For this review, take the finished solid that the model builds, in its own axes (mm). Face numbers are marked on the shaded views. A direction names the side the tool comes from. Coordinates: 2 decimals unless noted, no trailing zeros. Write each loop counter-clockwise with the first axis right and the second up, starting at its lowest first coordinate (ties: lowest second). Pieces come first, ordered by that corner, then holes.
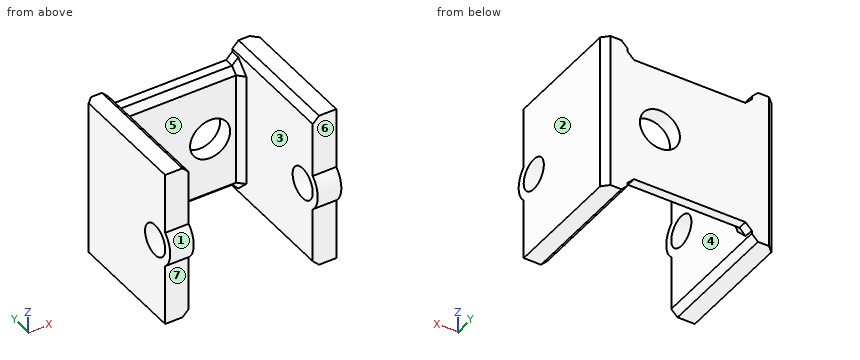
```python
from build123d import *

# Parameters (mm, degrees)
BOSS_EXTRUDE1_DEPTH            = 50
CUT_EXTRUDE1_DEPTH             = 67.839827199
CUT_EXTRUDE1_DEPTH_BACK        = 67.839827199
SKETCH3_W                      = 39.5
SKETCH3_H                      = 5
CHAMFER1_SIZE                  = 2
BOSS_EXTRUDE2_DEPTH            = 7.5
CUT_EXTRUDE4_REACH             = 86.085
SKETCH5_R                      = 5
CUT_EXTRUDE4_DIRECTION_2_DEPTH = 85.084778646
SKETCH6_R                      = 6.375
CUT_EXTRUDE5_DEPTH             = 69.182200757


with BuildPart() as part:
    # Sketch1 → Boss-Extrude1 (new body)
    with BuildSketch(Plane.XY):
        Polygon((-27.25, 0), (-19.75, 0), (-19.75, 35), (19.75, 35), (19.75, 0), (27.25, 0), (27.25, 40), (-27.25, 40), align=None)
    extrude(amount=BOSS_EXTRUDE1_DEPTH)

    # Sketch3 → Cut-Extrude1 (cut, two sides: drawn at the far end of the back side and taken through both)
    with BuildSketch(Plane(origin=(0, 35, 0), x_dir=(-1, 0, 0), z_dir=(0, -1, 0)).offset(-CUT_EXTRUDE1_DEPTH_BACK)):
        with Locations((0, -2.5)):
            Rectangle(SKETCH3_W, SKETCH3_H)
        with Locations((0, -47.5)):
            Rectangle(SKETCH3_W, SKETCH3_H)
    extrude(amount=CUT_EXTRUDE1_DEPTH + CUT_EXTRUDE1_DEPTH_BACK, mode=Mode.SUBTRACT)

    # Chamfer1
    chamfer1_edges = [part.edges().sort_by_distance(p)[0] for p in [
        (-19.75, 20, 0),
        (-19.75, 20, 50),
        (-27.25, 40, 25),
        (27.25, 40, 25),
        (19.75, 20, 50),
        (19.75, 35, 25),
        (-19.75, 35, 25),
        (-19.75, 37.5, 5),
        (0, 35, 5),
        (19.75, 37.5, 5),
        (19.75, 37.5, 45),
        (0, 35, 45),
        (-19.75, 37.5, 45),
        (19.75, 20, 0),
    ]]
    chamfer(chamfer1_edges, length=CHAMFER1_SIZE)

    # Sketch4 → Boss-Extrude2 (add)
    with BuildSketch(Plane.ZY.offset(27.25)):
        with BuildLine():
            Line((30.590169944, 0), (19.409830056, 0))
            ThreePointArc((19.409830056, 0), (25, -2.5), (30.590169944, 0))
        make_face()
    boss_extrude2 = extrude(amount=-BOSS_EXTRUDE2_DEPTH)

    # Sketch5 → Cut-Extrude4 (cut, up to next)
    with BuildSketch(Plane.ZY.offset(27.25), mode=Mode.PRIVATE) as cut_extrude4_sk1:
        with Locations(Location((25, 5, 0), (0, 0, 180))):
            Circle(SKETCH5_R)
    cut_extrude4_tool1 = extrude(cut_extrude4_sk1.sketch, amount=-CUT_EXTRUDE4_REACH, mode=Mode.PRIVATE) & part.part
    cut_extrude4 = cut_extrude4_tool1.solids().sort_by_distance((-27.25, 5, 25))[0]
    add(cut_extrude4, mode=Mode.SUBTRACT)

    # Sketch5 → Cut-Extrude4 direction 2 (cut)
    with BuildSketch(Plane.ZY.offset(27.25)):
        with Locations(Location((25, 5, 0), (0, 0, 180))):
            Circle(SKETCH5_R)
    cut_extrude4_direction_2 = extrude(amount=CUT_EXTRUDE4_DIRECTION_2_DEPTH, mode=Mode.SUBTRACT)

    # Mirror1: Boss-Extrude2, Cut-Extrude4, Cut-Extrude4 direction 2 across plane
    add(boss_extrude2.mirror(Plane(origin=(0, 0, 0), x_dir=(0, 0, 1), z_dir=(1, 0, 0))))
    add(cut_extrude4.mirror(Plane(origin=(0, 0, 0), x_dir=(0, 0, 1), z_dir=(1, 0, 0))), mode=Mode.SUBTRACT)
    add(cut_extrude4_direction_2.mirror(Plane(origin=(0, 0, 0), x_dir=(0, 0, 1), z_dir=(1, 0, 0))), mode=Mode.SUBTRACT)

    # Sketch6 → Cut-Extrude5 (cut, through all)
    with BuildSketch(Plane.XZ.offset(-35)):
        with Locations(Location((9.5, 25, 0), (0, 0, 270))):
            Circle(SKETCH6_R)
    extrude(amount=-CUT_EXTRUDE5_DEPTH, mode=Mode.SUBTRACT)


solid = part.part
```
Q1. For probe 1 along X at (y, z) = (10, 40); probe 2 along Y at (x, z) = (-23, 25), list the stretches that pass through material, from the lowest coordinate up.
Ans:
probe 1: x = -27.25 to -19.75, 19.75 to 27.25
probe 2: y = -2.5 to 0, 10 to 40
Q2. Add section C-C (y = 5). State the section outline as (x, z) points, then the cut area to 3 significant figures.
Ans:
outline: (-27.25, 0) - (-21.75, 0) - (-19.75, 2) - (-19.75, 20) - (-27.25, 20) - close; (-27.25, 30) - (-19.75, 30) - (-19.75, 48) - (-21.75, 50) - (-27.25, 50) - close; (19.75, 2) - (21.75, 0) - (27.25, 0) - (27.25, 20) - (19.75, 20) - close; (19.75, 30) - (27.25, 30) - (27.25, 50) - (21.75, 50) - (19.75, 48) - close
area: 592 mm2
Q3. Draft analysis for pull direction X (two halves, no side actions). For the marked faces 1, 2, 3 and 4, state which applies: +X half, -X half, draft (parallel to the pull), parting line (faces both ways), or undercut.
Ans:
face 1: draft
face 2: +X half
face 3: undercut
face 4: undercut
Q4. Add section D-D (z = 40). State the section outline as (x, y) points.
Ans:
outline: (-27.25, 0) - (-19.75, 0) - (-19.75, 33) - (-17.75, 35) - (17.75, 35) - (19.75, 33) - (19.75, 0) - (27.25, 0) - (27.25, 38) - (25.25, 40) - (-25.25, 40) - (-27.25, 38) - close
Q5. Clearance check with flat-ended pins moving along their axes: pin 1 Ø6 at (y, z) = (5, 25) entering from -X; pin 2 Ø10 at (x, z) = (-16, 16.5) entering from -Y; pin 3 Ø16 at (y, z) = (5, 25) entering from +X; pin 4 Ø2 at (x, z) = (-25, 45) entering from -Y. State where each tip first meets the part, or that it passes through.
Ans:
pin 1: passes through
pin 2: stops at y = -0.41
pin 3: stops at x = 27.25
pin 4: stops at y = 0
Q6. Add section B-B (x = 23.5). State the section outline as (y, z) points.
Ans:
outline: (0, 0) - (40, 0) - (40, 50) - (0, 50) - (0, 30.59) arc R7.5 ccw to (0, 19.41) - close; hole circle Ø10 at (5, 25)
Q7. Add section A-A (y = 13). State the section outline as (x, z) points.
Ans:
outline: (-27.25, 0) - (-21.75, 0) - (-19.75, 2) - (-19.75, 48) - (-21.75, 50) - (-27.25, 50) - close; (19.75, 2) - (21.75, 0) - (27.25, 0) - (27.25, 50) - (21.75, 50) - (19.75, 48) - close
Q8. Tool access review of the marked faces 5, 6 and 7: name each direction out of +Z, -Z, +X, -X, +Y, -Y from which nothing blocks a thin tool from reaching the whole face with its end or side.
Ans:
face 5: +Z, -Z, -Y
face 6: +Z, +X, -X, -Y
face 7: -Z, +X, -X, -Y
